Part model, mm, in its own coordinate system. A direction names the side the tool comes from. Coordinates: 2 decimals unless noted, no trailing zeros. Order: outer loops, then holes, each group sorted by start corner. A loop starts at its lowest first (then second) coordinate and runs counter-clockwise, first axis right, second up. Notation, with made-up numbers: (64, -7) - (81, -7) arc R23 cw to (81, 7) - close; hole circle Ø5 at (28, 85). An arc over 180 degrees is marked (long way). Use a Markdown table: item, result. Add a question column.
1) Wall check: L1, parallel to Y at x = 2.95, z = 5; L2, parallel to X at y = 8, z = 6.75; L3, parallel to Y at x = 2.15, z = 5. Give the ranges that are in metal, low to high. Write a range as [from, to].
2) Saw through at B-B on z = 4. List the corners of the cut face in (x, y).
3) Two-plate mould, pull along Z, no slides. Class faces 1 (the face through (0, -5, 0)), 2 (the face through (0, -5, 10)), 3 (the face through (0, -11.9, 6.2)), 4 (the face through (-6.39, -1.2, 4.93)): +Z half, -Z half, draft (parallel to the pull), parting line (faces both ways), or undercut.
4) Saw through at C-C on x = -3.5. List the corners of the cut face in (y, z), then the cut area to 3 significant figures.
5) Saw through at A-A on y = -11. List the corners of the cut face in (x, z).
6) Tool access for faces 5 (the face through (1.25, 6.7, 3.8)), 6 (the face through (4.25, 9.4, 3.8)), 7 (the face through (2, -14, 5)), 8 (the face through (-2, -14, 5)), 9 (the face through (-4.25, 6.7, 3.8)): list every direction of +Z, -Z, +X, -X, +Y, -Y with a clear straight run to the whole face (end or side of a thin tool).
7) Saw through at D-D on z = 2.25. List the corners of the cut face in (x, y), then the cut area to 3 significant figures.
8) Drop flat-ended pins along their axis: P1, Ø3, axis at y = 9, z = 4.5, coming from the -X side; P2, Ø3, axis at y = 7.5, z = 5.5, coming from the +X side; P3, Ø5, axis at y = -17, z = 5, coming from the +X side. Give the stop position or say it passes through.
```python
from build123d import *

# Parameters (mm, degrees)
BOSS_EXTRUDE1_DEPTH     = 10
SKETCH2_R               = 1.5
CUT_EXTRUDE1_DEPTH      = 3.25
CUT_EXTRUDE1_DEPTH_BACK = 11.75


with BuildPart() as part:
    # Sketch1 → Boss-Extrude1 (new body)
    with BuildSketch(Plane.XY):
        with BuildLine():
            ThreePointArc((2, -6.184658438), (0, -6.5), (-2, -6.184658438))
            Line((-2, -6.184658438), (-2, -21.5))
            Line((-2, -21.5), (2, -21.5))
            Line((2, -21.5), (2, -6.184658438))
        make_face()
        with BuildLine():
            Line((-2, -3.464101615), (-2, -6.184658438))
            ThreePointArc((-2, -6.184658438), (0, -6.5), (2, -6.184658438))
            Line((2, -6.184658438), (2, -3.464101615))
            ThreePointArc((2, -3.464101615), (0, -4), (-2, -3.464101615))
        make_face()
        with BuildLine():
            ThreePointArc((-1.25, 6.378675411), (-2.84531818, 5.844156436), (-4.25, 4.918078893))
            ThreePointArc((-4.25, 4.918078893), (-6.370503831, -1.290999975), (-2, -6.184658438))
            Line((-2, -6.184658438), (-2, -3.464101615))
            ThreePointArc((-2, -3.464101615), (-3.97884698, 0.410824427), (-1.25, 3.799671038))
            Line((-1.25, 3.799671038), (-1.25, 6.378675411))
        make_face()
        with BuildLine():
            ThreePointArc((4.25, 4.918078893), (2.84531818, 5.844156436), (1.25, 6.378675411))
            Line((1.25, 6.378675411), (1.25, 3.799671038))
            ThreePointArc((1.25, 3.799671038), (3.240370349, 2.34520788), (4, 0))
            ThreePointArc((4, 0), (3.464101615, -2), (2, -3.464101615))
            Line((2, -3.464101615), (2, -6.184658438))
            ThreePointArc((2, -6.184658438), (5.25594901, -3.824264635), (6.5, 0))
            ThreePointArc((6.5, 0), (5.910795209, 2.704163457), (4.25, 4.918078893))
        make_face()
        with BuildLine():
            Line((1.25, 11.168078893), (1.25, 6.378675411))
            ThreePointArc((1.25, 6.378675411), (2.84531818, 5.844156436), (4.25, 4.918078893))
            Line((4.25, 4.918078893), (4.25, 11.168078893))
            Line((4.25, 11.168078893), (1.25, 11.168078893))
        make_face()
        with BuildLine():
            Line((-4.25, 11.168078893), (-4.25, 4.918078893))
            ThreePointArc((-4.25, 4.918078893), (-2.84531818, 5.844156436), (-1.25, 6.378675411))
            Line((-1.25, 6.378675411), (-1.25, 11.168078893))
            Line((-1.25, 11.168078893), (-4.25, 11.168078893))
        make_face()
    extrude(amount=BOSS_EXTRUDE1_DEPTH)

    # Sketch2 → Cut-Extrude1 (cut, two sides)
    with BuildSketch(Plane(origin=(4.25, 0, 0), x_dir=(0, 0, -1), z_dir=(1, 0, 0))) as cut_extrude1_sk:
        with Locations((-5, 8.043078893)):
            Circle(SKETCH2_R)
        with Locations((-5, -17)):
            Circle(SKETCH2_R)
        with Locations((-5, -11)):
            Circle(SKETCH2_R)
    extrude(amount=CUT_EXTRUDE1_DEPTH, mode=Mode.SUBTRACT)
    extrude(cut_extrude1_sk.sketch, amount=-CUT_EXTRUDE1_DEPTH_BACK, mode=Mode.SUBTRACT)


solid = part.part
```
Results are:
| question | item | result |
|---|---|---|
| 1 | L1 | [-5.79, -2.7], [2.7, 6.54], [9.54, 11.17] |
| 1 | L2 | [-4.25, -1.25], [1.25, 4.25] |
| 1 | L3 | [-6.13, -3.37], [3.37, 6.54], [9.54, 11.17] |
| 2 | outline | (-4.25, 4.92) arc R6.5 ccw to (-2, -6.18) - (-2, -9.88) - (2, -9.88) - (2, -6.18) arc R6.5 ccw to (4.25, 4.92) - (4.25, 6.93) - (1.25, 6.93) - (1.25, 3.8) arc R4 cw (long way) to (-1.25, 3.8) - (-1.25, 6.93) - (-4.25, 6.93) - close; (-4.25, 9.16) - (-1.25, 9.16) - (-1.25, 11.17) - (-4.25, 11.17) - close; (-2, -21.5) - (2, -21.5) - (2, -18.12) - (-2, -18.12) - close; (-2, -15.88) - (2, -15.88) - (2, -12.12) - (-2, -12.12) - close; (1.25, 9.16) - (4.25, 9.16) - (4.25, 11.17) - (1.25, 11.17) - close |
| 3 | face 1 | -Z half |
| 3 | face 2 | +Z half |
| 3 | face 3 | undercut |
| 3 | face 4 | draft |
| 4 | outline | (-5.48, 0) - (-1.94, 0) - (-1.94, 10) - (-5.48, 10) - close; (1.94, 0) - (11.17, 0) - (11.17, 10) - (1.94, 10) - close; hole circle Ø3 at (8.04, 5) |
| 4 | area | 121 mm2 |
| 5 | outline | (-2, 0) - (2, 0) - (2, 3.5) - (-2, 3.5) - close; (-2, 6.5) - (2, 6.5) - (2, 10) - (-2, 10) - close |
| 6 | face 5 | +Z, -Z, +Y |
| 6 | face 6 | +Z, -Z, +X, +Y |
| 6 | face 7 | +Z, -Z, +X, -Y |
| 6 | face 8 | +Z, -Z, -X, -Y |
| 6 | face 9 | +Z, -Z, -X, +Y |
| 7 | outline | (-4.25, 4.92) arc R6.5 ccw to (-2, -6.18) - (-2, -21.5) - (2, -21.5) - (2, -6.18) arc R6.5 ccw to (4.25, 4.92) - (4.25, 11.17) - (1.25, 11.17) - (1.25, 3.8) arc R4 cw (long way) to (-1.25, 3.8) - (-1.25, 11.17) - (-4.25, 11.17) - close |
| 7 | area | 169 mm2 |
| 8 | P1 | x = -4.25 |
| 8 | P2 | x = 4.25 |
| 8 | P3 | x = 2 |
